from build123d import *

# Parameters (mm, degrees)
CROQUIS1_W              = 54
CROQUIS1_H              = 13
SALIENTE_EXTRUIR1_DEPTH = 10
CORTAR_EXTRUIR1_DEPTH   = 8
CROQUIS1_4_R            = 2.875
CORTAR_EXTRUIR2_DEPTH   = 11


with BuildPart() as part:
    # Croquis1 → Saliente-Extruir1 (new body)
    with BuildSketch(Plane(origin=(0, 0, 0), x_dir=(1, 0, 0), z_dir=(0, 1, 0))):
        Rectangle(CROQUIS1_W, CROQUIS1_H)
    extrude(amount=SALIENTE_EXTRUIR1_DEPTH)

    # Croquis1<3> → Cortar-Extruir1 (cut)
    with BuildSketch(Plane(origin=(0, 0, 0), x_dir=(1, 0, 0), z_dir=(0, 1, 0))):
        Polygon((-18.33826859, -4.05), (-13.66173141, -4.05), (-11.32346282, 0), (-13.66173141, 4.05), (-18.33826859, 4.05), (-20.67653718, 0), align=None)
        Polygon((20.67653718, 0), (18.33826859, 4.05), (13.66173141, 4.05), (11.32346282, 0), (13.66173141, -4.05), (18.33826859, -4.05), align=None)
    extrude(amount=CORTAR_EXTRUIR1_DEPTH, mode=Mode.SUBTRACT)

    # Croquis1<4> → Cortar-Extruir2 (cut, through all)
    with BuildSketch(Plane(origin=(0, 0, 0), x_dir=(1, 0, 0), z_dir=(0, 1, 0))):
        with Locations((-16, 0)):
            Circle(CROQUIS1_4_R)
        with Locations((16, 0)):
            Circle(CROQUIS1_4_R)
    extrude(amount=CORTAR_EXTRUIR2_DEPTH, mode=Mode.SUBTRACT)


solid = part.part
Source: CAD feature listing. Evaluate the final solid. Frame: model axes, mm. A direction names the side the tool comes from. Give positions to 0.01 mm unless a question says otherwise; leave off trailing zeros. Write each loop counter-clockwise with the first axis right and the second up, starting at its lowest first coordinate (ties: lowest second). Pieces come first, ordered by that corner, then holes. Notation, with made-up numbers: M 0,35.25 L 31,35.25 A21 cw 31,70.25 Z; hole C 37.25,46.5 d11. An arc over 180 degrees is marked long. Answer as a JSON object with one key per item and string values.
Q1. Contact query for flat-ended pins moving along their axis: P1, Ø6.5, axis at x = -16, z = 0, coming from the +Y side; P2, Ø4, axis at x = 15, z = 1.5, coming from the -Y side. Output: stop coordinate, or through.
Geometry check:
{"P1": "stops at y = 10", "P2": "stops at y = 8"}
Q2. Cut plane B-B, the plane x = -16. Return the cut outline in (y, z) (3 decimals).
Geometry check:
{"outline": "M 0,-6.5 L 10,-6.5 L 10,-2.875 L 8,-2.875 L 8,-4.05 L 0,-4.05 Z; M 0,4.05 L 8,4.05 L 8,2.875 L 10,2.875 L 10,6.5 L 0,6.5 Z"}
Q3. Cut plane D-D, the plane z = -1.75. Return the cut outline in (x, y), then the cut area to 3 significant figures.
Geometry check:
{"outline": "M -27,0 L -19.67,0 L -19.67,8 L -18.28,8 L -18.28,10 L -27,10 Z; M -13.72,8 L -12.33,8 L -12.33,0 L 12.33,0 L 12.33,8 L 13.72,8 L 13.72,10 L -13.72,10 Z; M 18.28,8 L 19.67,8 L 19.67,0 L 27,0 L 27,10 L 18.28,10 Z", "area": "404 mm^2"}
Q4. Ray query, line 1 along Z through (x, y) = (14, 5.75); line 2 along X through (y, z) = (7.25, 2.75); line 3 along X through (y, z) = (3.75, -0.75). Return the intervals inside material, ascending.
Geometry check:
{"line 1": "z = -6.5 to -4.05, 4.05 to 6.5", "line 2": "x = -27 to -19.09, -12.91 to 12.91, 19.09 to 27", "line 3": "x = -27 to -20.24, -11.76 to 11.76, 20.24 to 27"}
Q5. Cut plane C-C, the plane y = 8.5. Return the cut outline in (x, z) (3 decimals), then the cut area to 3 significant figures.
Geometry check:
{"outline": "M -27,-6.5 L 27,-6.5 L 27,6.5 L -27,6.5 Z; hole C -16,0 d5.75; hole C 16,0 d5.75", "area": "650 mm^2"}
Q6. Cut plane A-A, the plane z = 0.5. Return the cut outline in (x, y).
Geometry check:
{"outline": "M -27,0 L -20.39,0 L -20.39,8 L -18.83,8 L -18.83,10 L -27,10 Z; M -13.17,8 L -11.61,8 L -11.61,0 L 11.61,0 L 11.61,8 L 13.17,8 L 13.17,10 L -13.17,10 Z; M 18.83,8 L 20.39,8 L 20.39,0 L 27,0 L 27,10 L 18.83,10 Z"}
Q7. Access query for faces 1 (the face through (16, 4, -4.05)), 2 (the face through (-13.258, 8.986, -0.864)). Directions: +Z, -Z, +X, -X, +Y, -Y. A direction counts if a zero-diameter tool reaches every point of the face in a straight line with its end or side. Return the directions, or none.
Geometry check:
{"face 1": "-Y", "face 2": "+Y, -Y"}
Q8. Mould query, pull axis X, two halves, no side actions, for faces 3 (the face through (-27, 5, 0)), 4 (the face through (18.656, 8.986, 1.101)), 5 (the face through (0, 5, 6.5)). Classes: +X half, -X half, draft (parallel to the pull), parting line (faces both ways), or undercut.
Geometry check:
{"face 3": "-X half", "face 4": "undercut", "face 5": "draft"}
